Job drawing, mm, ordinate dimensions from the low corner. One solid piece. A direction names the side the tool comes from. Give positions to 0.01 mm unless a question says otherwise; leave off trailing zeros. Write each loop counter-clockwise with the first axis right and the second up, starting at its lowest first coordinate (ties: lowest second). Pieces come first, ordered by that corner, then holes. Notation, with made-up numbers: (-4, 24.5) - (55, 24.5) arc R19 cw to (55, 46.5) - close; hole circle Ø4 at (26, 18). An arc over 180 degrees is marked (long way). Answer in a Markdown table with one row per item. Add a question column.
1. Pull direction X, two halves, no side cores. Call the marked faces 4, 5, 6 and 7: released by +X, released by -X, zero draft, split by the parting line, or undercut.
2. Band-saw the part on C-C on z = 5.5. Write the cut outline in (x, y) (3 decimals).
3. Band-saw the part on D-D on x = 14.25. Write the cut outline in (y, z) (3 decimals).
4. Band-saw the part on B-B on y = 13.25. Write the cut outline in (x, z), plus the area to 4 significant figures.
5. Which spindle directions (+Z, -Z, +X, -X, +Y, -Y) get a long thin tool onto all of the face, cutting with end or side? Do the marked faces 1, 2 and 3. Say none if no direction does.
6. Band-saw the part on A-A on x = 9. Write the cut outline in (y, z) (3 decimals).
7. Drop flat-ended pins along their axis: pin 1 Ø5 at (y, z) = (12.5, 5) entering from +X; pin 2 Ø1.5 at (x, y) = (16, 11.5) entering from -Z; pin 3 Ø0.9 at (x, z) = (16, 9.5) entering from +Y; pin 4 Ø1.6 at (y, z) = (7.5, 11.5) entering from -X. Give the stop position or say it passes through.
8. Probe line 1 along Y through (x, z) = (9, 12.05) (3 decimals); line 2 along Y through (x, z) = (9, 11.05) (3 decimals); line 3 along Z through (x, y) = (12, 10.25). List the from-to ranges inside material, lowest first.
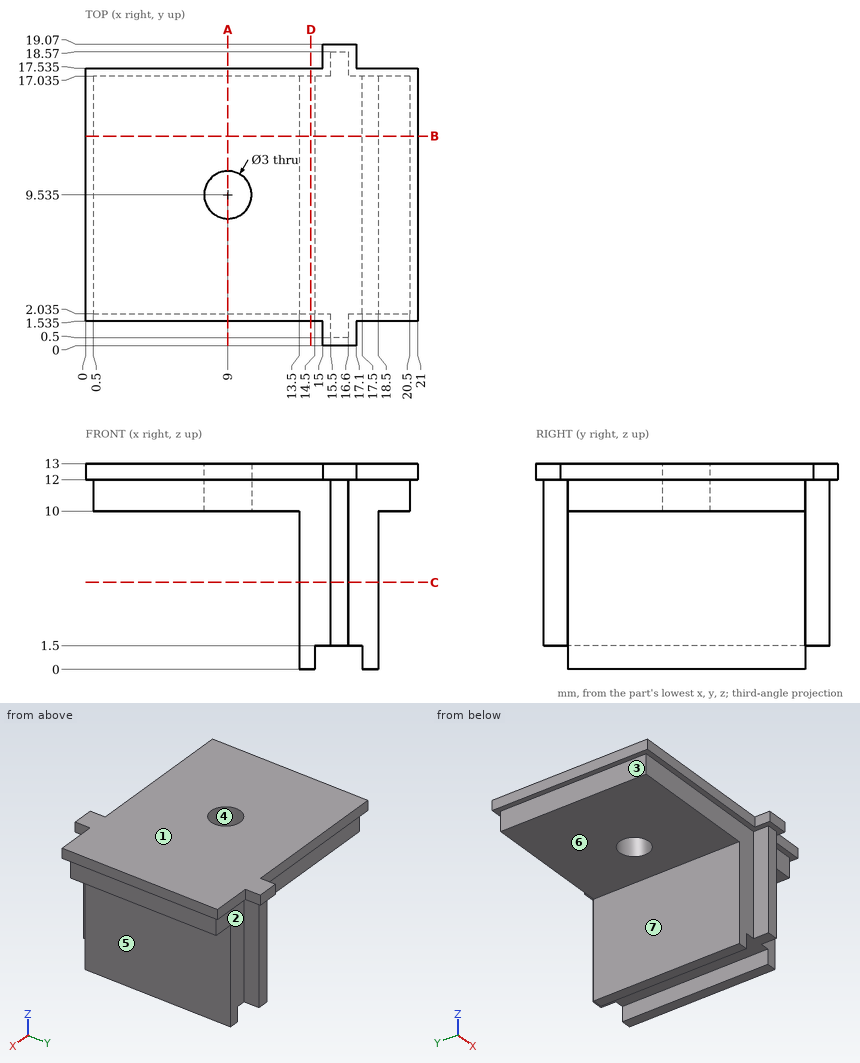
Values:
| question | item | result |
|---|---|---|
| 1 | face 4 | undercut |
| 1 | face 5 | released by +X |
| 1 | face 6 | zero draft |
| 1 | face 7 | released by -X |
| 2 | outline | (13.5, 2.035) - (15.5, 2.035) - (15.5, 0.5) - (16.6, 0.5) - (16.6, 2.035) - (18.5, 2.035) - (18.5, 17.035) - (16.6, 17.035) - (16.6, 18.57) - (15.5, 18.57) - (15.5, 17.035) - (13.5, 17.035) - close |
| 3 | outline | (1.535, 12) - (2.035, 12) - (2.035, 0) - (17.035, 0) - (17.035, 12) - (17.535, 12) - (17.535, 13) - (1.535, 13) - close |
| 4 | outline | (0, 12) - (0.5, 12) - (0.5, 10) - (13.5, 10) - (13.5, 0) - (14.5, 0) - (14.5, 1.5) - (17.5, 1.5) - (17.5, 0) - (18.5, 0) - (18.5, 10) - (20.5, 10) - (20.5, 12) - (21, 12) - (21, 13) - (0, 13) - close |
| 4 | area | 106.5 mm² |
| 5 | face 1 | +Z, +X, -X, +Y, -Y |
| 5 | face 2 | -Z, +X, +Y |
| 5 | face 3 | -Z, -X, +Y, -Y |
| 6 | outline | (1.535, 12) - (2.035, 12) - (2.035, 10) - (8.035, 10) - (8.035, 13) - (1.535, 13) - close; (11.035, 10) - (17.035, 10) - (17.035, 12) - (17.535, 12) - (17.535, 13) - (11.035, 13) - close |
| 7 | pin 1 | stops at x = 18.5 |
| 7 | pin 2 | stops at z = 1.5 |
| 7 | pin 3 | stops at y = 18.57 |
| 7 | pin 4 | stops at x = 0 |
| 8 | line 1 | y = 1.535 to 8.035, 11.035 to 17.535 |
| 8 | line 2 | y = 2.035 to 8.035, 11.035 to 17.035 |
| 8 | line 3 | z = 10 to 13 |
